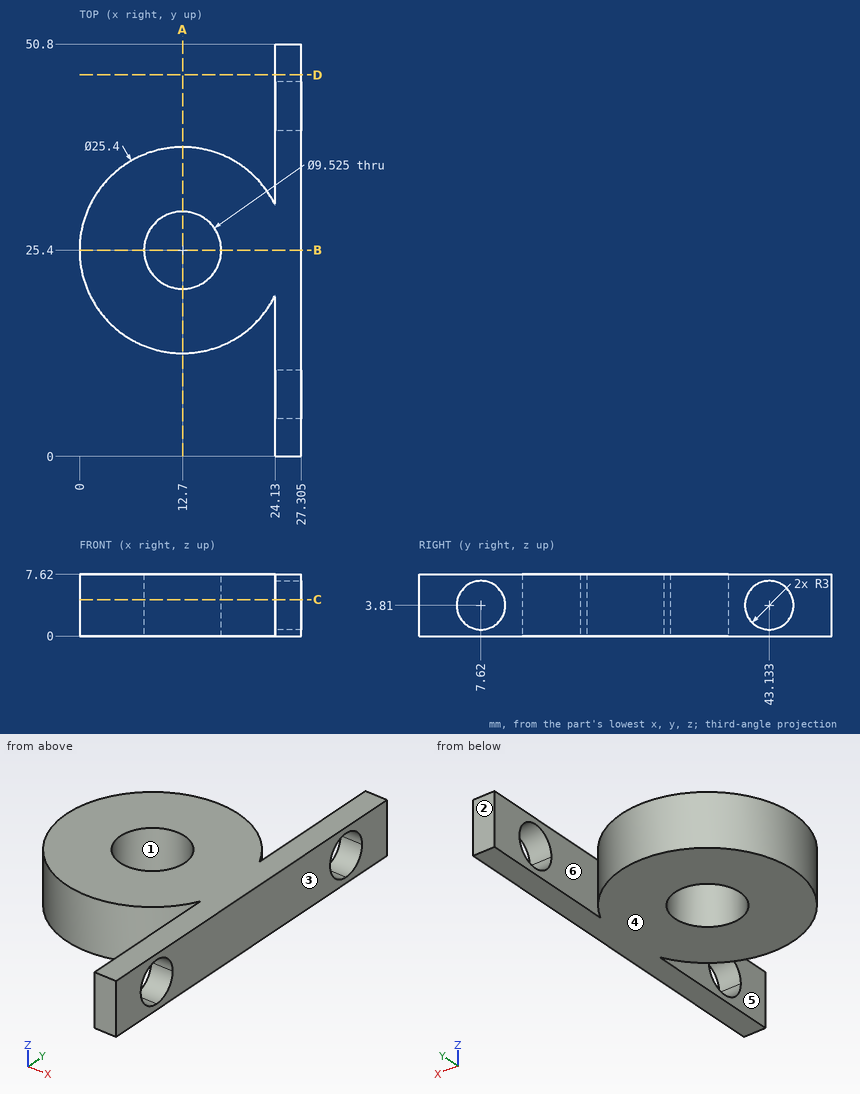
The figure shows three views and two pictorial views of one solid part (mm, origin at its lowest corner). Answer the questions. A direction names the side the tool comes from. Round coordinates to 2 decimals unless told otherwise and drop trailing zeros. Write each loop counter-clockwise with the first axis right and the second up, starting at its lowest first coordinate (ties: lowest second). Pieces come first, ordered by that corner, then holes. Notation, with made-up numbers: M 9.5,78.5 L 34.5,78.5 A14 cw 34.5,98.5 Z; hole C 13.5,38.5 d10. An arc over 180 degrees is marked long. Write each question's results on one line, items separated by ' | '. Start each with the question number.
(1) The part is cut by section C-C, the plane z = 4.5. Write down the section's boundary in (x, y) (1 decimal).
(2) Determine the mould class of the marked faces 1, 2 and 3 for opening direction X: +X half, -X half, draft (parallel to the pull), parting line (faces both ways), or undercut.
(3) For the marked faces 4, 5 and 6, determine the directions among +Z, -Z, +X, -X, +Y, -Y from which every point of the face is accessible in a straight line to the end or side of a thin tool.
(4) The part is cut by section B-B, the plane y = 25.4. Write down the section's boundary in (x, z) (1 decimal).
(5) Find the intervals of material crossed by line 1 (Y direction, x = 12.7, z = 2.75); line 2 (Y direction, x = 24.75, z = 1.25) (1 decimal); line 3 (X direction, y = 40, z = 1.75) (1 decimal), in increasing order.
(6) The part is cut by section D-D, the plane y = 47. Write down the section's boundary in (x, z) (1 decimal), and give its area (3 significant figures).
(7) Each of these flat-tipped pins is pushed along its axis until it touches: P1, Ø7.5, axis at x = 12.7, y = 25.4, coming from the +Z side; P2, Ø3, axis at y = 6.5, z = 2.5, coming from the +X side (3 decimals); P3, Ø3, axis at x = 20, z = 4, coming from the +Y side; P4, Ø2.5, axis at y = 5.5, z = 2.5, coming from the -X side. Where does it stop, or does it pass through?
(8) The part is cut by section A-A, the plane x = 12.7. Write down the section's boundary in (y, z).
Worked answers:
1) outline: M 24.1,0 L 27.3,0 L 27.3,4.7 L 24.1,4.7 Z; M 24.1,10.5 L 27.3,10.5 L 27.3,40.2 L 24.1,40.2 L 24.1,30.9 A12.7 ccw long 24.1,19.9 Z; M 24.1,46.1 L 27.3,46.1 L 27.3,50.8 L 24.1,50.8 Z; hole C 12.7,25.4 d9.5
2) face 1: undercut | face 2: draft | face 3: +X half
3) face 4: -Z, +X, -X, +Y, -Y | face 5: +Z, -Z, -Y | face 6: +Z, -Z, +Y
4) outline: M 0,0 L 7.9,0 L 7.9,7.6 L 0,7.6 Z; M 17.5,0 L 27.3,0 L 27.3,7.6 L 17.5,7.6 Z
5) line 1: y = 12.7 to 20.64, 30.16 to 38.1 | line 2: y = 0 to 6.1, 9.2 to 41.6, 44.7 to 50.8 | line 3: x = 24.1 to 27.3
6) outline: M 24.1,0 L 27.3,0 L 27.3,7.6 L 24.1,7.6 Z | area: 24.2 mm²
7) P1: passes through | P2: stops at x = 27.305 | P3: stops at y = 36.7 | P4: stops at x = 24.13
8) outline: M 12.7,0 L 20.64,0 L 20.64,7.62 L 12.7,7.62 Z; M 30.16,0 L 38.1,0 L 38.1,7.62 L 30.16,7.62 Z
